Geometry check sheet. Reference: the model listing, model coordinates, mm. Face numbers are marked on the shaded views. A direction names the side the tool comes from. Coordinates: 2 decimals unless noted, no trailing zeros. Loops run counter-clockwise (first coordinate to the right, second up) from the corner with the lowest first, then second, coordinate; pieces in that order, holes last.
from build123d import *

# Parameters (mm, degrees)
BOSS_EXTRUDE1_DEPTH = 45.72
SKETCH2_R           = 3.175
CUT_EXTRUDE1_DEPTH  = 59.143257563
SKETCH4_R           = 6.35
CUT_EXTRUDE2_DEPTH  = 19.05


with BuildPart() as part:
    # Sketch1 → Boss-Extrude1 (new body)
    with BuildSketch(Plane.XY):
        Polygon((-4.745410922, 25.4), (-25.4, 4.745410922), (-25.4, 0), (0, 0), (0, 25.4), align=None)
        Polygon((-4.826, 18.49441627), (-4.826, 4.826), (-18.49441627, 4.826), align=None, mode=Mode.SUBTRACT)
    extrude(amount=BOSS_EXTRUDE1_DEPTH)

    # Sketch2 → Cut-Extrude1 (cut, through all)
    with BuildSketch(Plane.XZ):
        with Locations(Location((-12.7, 35.56, 0), (0, 0, 270))):
            Circle(SKETCH2_R)
        with Locations(Location((-12.7, 10.16, 0), (0, 0, 270))):
            Circle(SKETCH2_R)
    extrude(amount=-CUT_EXTRUDE1_DEPTH, mode=Mode.SUBTRACT)

    # Sketch4 → Cut-Extrude2 (cut)
    with BuildSketch(Plane(origin=(0, 25.4, 0), x_dir=(1, 0, 0), z_dir=(0, 1, 0))):
        with Locations(Location((-12.7, -10.16, 0), (0, 0, 227.739186389))):
            Circle(SKETCH4_R)
        with Locations(Location((-12.7, -35.56, 0), (0, 0, 227.739186389))):
            Circle(SKETCH4_R)
    extrude(amount=-CUT_EXTRUDE2_DEPTH, mode=Mode.SUBTRACT)


solid = part.part
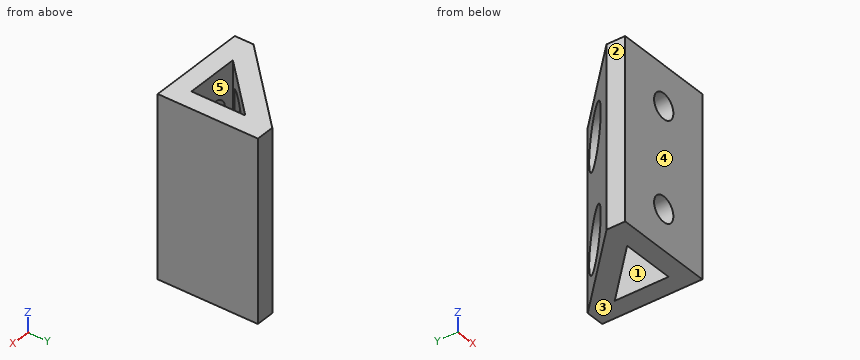
(1) Sectioned sample at A-A on z = 25. Record the cut outline in (x, y), and give its area (3 significant figures).
Findings:
outline: (-25.4, 0) - (0, 0) - (0, 25.4) - (-4.75, 25.4) - (-25.4, 4.75) - close; hole (-18.49, 4.83) - (-4.83, 4.83) - (-4.83, 18.49) - close
area: 338 mm2
(2) Scan lines: L1, parallel to Z at x = -12.7, y = 17; L2, parallel to Z at x = -11, y = 2.75; L3, parallel to X at y = 3.65, z = 10.16 (3 decimals). Record each from-to range of solid material in increasing order.
Findings:
L1: z = 0 to 3.81, 16.51 to 29.21, 41.91 to 45.72
L2: z = 0 to 7.48, 12.84 to 32.88, 38.24 to 45.72
L3: x = -25.4 to -15.875, -9.525 to 0
(3) Access from +Z, -Z, +X, -X, +Y, -Y to the whole of each face (thin tool, end or side, straight path). Record for the marked faces 1 and 2.
Findings:
face 1: +Z, -Z
face 2: +Z, -Z, -X, +Y, -Y
(4) Gauge pin test, flat ends, axial feed: pin 1 Ø0.6 at (x, z) = (-18, 12) entering from +Y; pin 2 Ø2 at (y, z) = (6, 21.5) entering from -X; pin 3 Ø4 at (x, z) = (-9, 13) entering from +Y. Record the tip position at first contact, or that the pin passes through.
Findings:
pin 1: stops at y = 6.35
pin 2: stops at x = -25.15
pin 3: stops at y = 23.15
(5) Sectioned sample at C-C on x = -12.7. Record the cut outline in (y, z) (3 decimals), and give its area (3 significant figures).
Findings:
outline: (0, 0) - (4.826, 0) - (4.826, 6.985) - (0, 6.985) - close; (0, 13.335) - (4.826, 13.335) - (4.826, 32.385) - (0, 32.385) - close; (0, 38.735) - (4.826, 38.735) - (4.826, 45.72) - (0, 45.72) - close; (10.62, 0) - (17.445, 0) - (17.445, 3.81) - (10.62, 3.81) - close; (10.62, 16.51) - (17.445, 16.51) - (17.445, 29.21) - (10.62, 29.21) - close; (10.62, 41.91) - (17.445, 41.91) - (17.445, 45.72) - (10.62, 45.72) - close
area: 298 mm2
(6) Sectioned sample at D-D on z = 35.56. Record the cut outline in (x, y) (3 decimals).
Findings:
outline: (-25.4, 0) - (-15.875, 0) - (-15.875, 4.826) - (-18.494, 4.826) - (-16.97, 6.35) - (-19.05, 6.35) - (-19.05, 11.095) - (-25.4, 4.745) - close; (-9.525, 0) - (0, 0) - (0, 25.4) - (-4.745, 25.4) - (-6.35, 23.795) - (-6.35, 16.97) - (-4.826, 18.494) - (-4.826, 4.826) - (-9.525, 4.826) - close
(7) Sectioned sample at B-B on y = 17.75. Record the cut outline in (x, z), and give its area (3 significant figures).
Findings:
outline: (-12.4, 0) - (-5.57, 0) - (-5.57, 45.72) - (-12.4, 45.72) - (-12.4, 41.9) arc R6.35 cw to (-12.4, 29.22) - (-12.4, 16.5) arc R6.35 cw to (-12.4, 3.82) - close; (-4.83, 0) - (0, 0) - (0, 45.72) - (-4.83, 45.72) - close
area: 414 mm2
(8) Draft check along Y on the marked faces 3, 4 and 5. Enter one of: +Y half, -Y half, draft (parallel to the pull), parting line (faces both ways), or undercut.
Findings:
face 3: draft
face 4: -Y half
face 5: undercut
